Autodesk Inventor part; units mm, degrees
ref_plane "YZ Plane" through (0, 0, 0) normal (1, 0, 0) x (0, 1, 0)
ref_plane "XZ Plane" through (0, 0, 0) normal (0, 1, 0) x (-1, 0, 0)
ref_plane "XY Plane" through (0, 0, 0) normal (0, 0, 1) x (1, 0, 0)
sketch "Sketch1" plane through (0, 0, 0) normal (0, 1, 0) x (-1, 0, 0)
  circle A0 centre (0, 0) radius 11
  circle A1 centre (0, 0) radius 15
  circle A2 centre (0, 60) radius 7.5
  circle A3 centre (-45, 0) radius 7.5
  line L0 (0, 60) -> (0, 0)
  line L1 (0, 0) -> (-45, 0)
  line L2 (7.4412, 60.9375) -> (14.8824, 1.875)
  line L3 (-14.8824, 1.875) -> (-7.4412, 60.9375)
  line L4 (-2.5, 14.7902) -> (-46.25, 7.3951)
  line L5 (-2.5, -14.7902) -> (-46.25, -7.3951)
  circle A4 centre (0, 60) radius 2.5
  circle A5 centre (-45, 0) radius 2.5
  point P0 (-13.4892, 12.9327)
  dimension "d0" = 22
  dimension "d1" = 30
  dimension "d2" = 15
  dimension "d3" = 15
  dimension "d4" = 45
  dimension "d5" = 60
  dimension "d6" = 5
  dimension "d7" = 5
extrude "Extrusion1" add sketch "Sketch1" along normal blind 7 contours A0 L0 A1 L1 | A0 L1 A1 L0 | L0 A2 L2 A1 | A1 L4 L3 A2 L0 | L1 A3 L4 L3 A1 | A1 L5 A3 L1 | A1 L3 L4 | A2 | A3
fillet "Fillet1" radius 6 1 edges at (13.4892, 3.5, 12.9327)
properties part number "BellCrank"
Check sheet for the modelled part. Datum: model origin and axes. Units: mm. Round coordinates to 2 decimals unless told otherwise and drop trailing zeros. Loops run counter-clockwise (first coordinate to the right, second up) from the corner with the lowest first, then second, coordinate; pieces in that order, holes last. Notation, with made-up numbers: (-37.75, 11.5) - (-30.75, 11.5) arc R24 ccw to (-30.75, 40.5) - close; hole circle Ø1 at (74, -16). An arc over 180 degrees is marked (long way). Write item = value, one per line. Start each with the question number.
Q1. Thickness scan on L1, parallel to Z at x = 0, y = 4; L2, parallel to Z at x = 0.5, y = 2; L3, parallel to X at y = 2.25, z = 0.5. Record the ranges inside material, lowest first.
Q2. Release check for a two-part mould opening along Z. For faces 1 (the face through (-1.34, 3.45, 57.89)), 2 (the face through (12, 0, 18)), 3 (the face through (-11.11, 3.45, 31.82)) record: pulls with the +Z half, pulls with the -Z half, needs draft (parallel to the pull), parting line crosses it, or undercut.
Q3. Section check D-D (y = 4). Count the separate pieces of the cut face and the enclosed holes in it, plus the area to 3 significant figures.
Q4. Depth check by flat-ended pin: P1, Ø1.5, axis at y = 3.5, z = 42.5, coming from the +X side; P2, Ø3, axis at x = 18, y = 1.5, coming from the +Z side; P3, Ø3, axis at x = 35, y = 5, coming from the +Z side. Enter the tip coordinate at first touch or a pass-through.
Q5. Section check B-B (x = 0). Record the boundary of the cut face in (y, z).
Q6. Section check A-A (z = 4). Record the boundary of the cut face in (x, y).
Q7. Section check C-C (x = 45). Record the boundary of the cut face in (y, z), plus the area to 3 significant figures.
Derived:
q1.L1 = -15 to -11, 11 to 57.5, 62.5 to 67.5
q1.L2 = -14.99 to -10.99, 10.99 to 57.55, 62.45 to 67.48
q1.L3 = -14.99 to -10.99, 10.99 to 42.55, 47.45 to 52.48
q2.face_1 = undercut
q2.face_2 = needs draft
q2.face_3 = pulls with the +Z half
q3.separate_pieces = 1
q3.enclosed_holes = 3
q3.area = 2,120 mm^2
q4.P1 = 9.86
q4.P2 = 12.6
q4.P3 = 9.55
q5.outline = (0, -15) - (7, -15) - (7, -11) - (0, -11) - close; (0, 11) - (7, 11) - (7, 57.5) - (0, 57.5) - close; (0, 62.5) - (7, 62.5) - (7, 67.5) - (0, 67.5) - close
q6.outline = (-14.61, 0) - (-10.25, 0) - (-10.25, 7) - (-14.61, 7) - close; (10.25, 0) - (51.34, 0) - (51.34, 7) - (10.25, 7) - close
q7.outline = (0, -7.61) - (7, -7.61) - (7, -2.5) - (0, -2.5) - close; (0, 2.5) - (7, 2.5) - (7, 7.61) - (0, 7.61) - close
q7.area = 71.5 mm^2
